Autodesk Inventor part; units mm, degrees
ref_plane "YZ Plane" through (0, 0, 0) normal (1, 0, 0) x (0, 1, 0)
ref_plane "XZ Plane" through (0, 0, 0) normal (0, 1, 0) x (-1, 0, 0)
ref_plane "XY Plane" through (0, 0, 0) normal (0, 0, 1) x (1, 0, 0)
sketch "Sketch1" plane through (0, 0, 0) normal (0, 0, 1) x (1, 0, 0)
  circle A0 centre (0, 0) radius 152.4
  circle A1 centre (0, 0) radius 146.05
  dimension "d0" = 304.8
  dimension "d1" = 292.1
extrude "Extrusion1" add sketch "Sketch1" along normal blind 101.6
sketch "Sketch2" plane through (0, 0, 101.6) normal (0, 0, 1) x (1, 0, 0)
  circle A0 centre (0, 0) radius 146.05
  circle A1 centre (0, 0) radius 152.4
  line L0 (0, -146.05) -> (0, -152.4)
  line L1 (0, 146.05) -> (0, 152.4)
extrude "Extrusion3" cut sketch "Sketch2" against normal blind 38.1 contours A0 L0 A1 L1 picked at (-148.0019, 0)
ref_plane "Work Plane1" through (152.4, 0, 0) normal (-1, 0, 0) x (0, -1, 0)
sketch "Sketch3" plane through (152.4, 0, 0) normal (-1, 0, 0) x (0, -1, 0)
  line L0 (-4.7625, 101.6) -> (-4.7625, 76.2)
  line L1 (-4.7625, 76.2) -> (-23.8125, 76.2)
  line L2 (-23.8125, 76.2) -> (-23.8125, 101.6)
  line L3 (-23.8125, 101.6) -> (-4.7625, 101.6)
  line L4 (-152.4, 0) -> (152.4, 0)
  point P0 (0, 0)
  dimension "d8" = 25.4
  dimension "d9" = 19.05
  dimension "d10" = 4.7625
  dimension "d11" = 101.6
extrude "Extrusion4" cut sketch "Sketch3" along normal blind 38.1
properties part number "Bucketr" material "Polycarbonate, Clear"
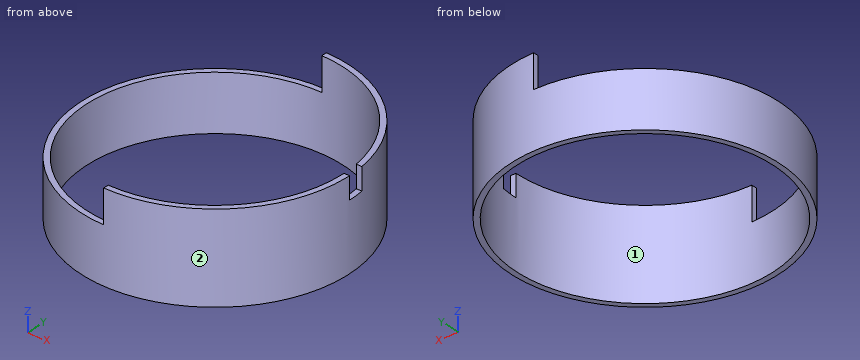
CAD build for the part. Positions are in the model's coordinates, mm. Face numbers are marked on the shaded views. Give positions to 0.01 mm unless a question says otherwise; leave off trailing zeros. Loops run counter-clockwise (first coordinate to the right, second up) from the corner with the lowest first, then second, coordinate; pieces in that order, holes last. Notation, with made-up numbers: M 46.5,86 L 95.5,86 A15 cw 95.5,105 Z; hole C 78.5,-34 d6. An arc over 180 degrees is marked long. Use one line per item in the form item = value.
Item 1: Slice it at A-A (z = 92). List the corners of the cut face in (x, y).
Determined:
outline = M 0,-152.4 A152.4 ccw 152.33,4.76 L 145.97,4.76 A146.05 cw 0,-146.05 Z; M 0,146.05 A146.05 cw 144.1,23.81 L 150.53,23.81 A152.4 ccw 0,152.4 Z
Item 2: Drill centre lines: probe 1 along X at (y, z) = (0, 49); probe 2 along X at (y, z) = (-5, 59). Where is each one in solid material? Low to high. Write a range as from..to.
Determined:
probe_1 = -152.4..-146.05, 146.05..152.4
probe_2 = -152.32..-145.96, 145.96..152.32
Item 3: Slice it at C-C (z = 47). List the corners of the cut face in (x, y), plus the area to 3 significant figures.
Determined:
outline = C 0,0 d304.8; hole C 0,0 d292.1
area = 5,950 mm2
Item 4: Slice it at B-B (y = 0). List the corners of the cut face in (x, z), plus the area to 3 significant figures.
Determined:
outline = M -152.4,0 L -146.05,0 L -146.05,63.5 L -152.4,63.5 Z; M 146.05,0 L 152.4,0 L 152.4,101.6 L 146.05,101.6 Z
area = 1,050 mm2
Item 5: Flat gauge pins, fed straight in: pin 1 (12 mm diameter, centred on y = -16, z = 72.5, fed in from -X); pin 2 (5 mm diameter, centred on y = -36, z = 49, fed in from -X); pin 3 (7 mm diameter, centred on y = -148.5, z = 74, fed in from -X). Where does each tip first touch, or does it go through?
Determined:
pin_1 = 144.38
pin_2 = -148.67
pin_3 = 0
Item 6: Two-plate mould, pull along X, no slides. Class the marked faces 1 and 2: pulls with the +X half, pulls with the -X half, needs draft (parallel to the pull), parting line crosses it, or undercut.
Determined:
face_1 = undercut
face_2 = parting line crosses it
